Read the model definition and answer for the solid it produces. Units are mm, in the model's axes. Face numbers are marked on the shaded views. A direction names the side the tool comes from. Coordinates: 2 decimals unless noted, no trailing zeros. Write each loop counter-clockwise with the first axis right and the second up, starting at its lowest first coordinate (ties: lowest second). Pieces come first, ordered by that corner, then holes.
1) Find the intervals of material crossed by line 1 (Y direction, x = -29, z = 3.35); line 2 (Y direction, x = -24, z = 1.8); line 3 (X direction, y = -20, z = 1.9), in increasing order.
2) The part is cut by section D-D (x = -33). Determine the outline of the cut face in (y, z).
3) The part is cut by section A-A (x = -24). Determine the outline of the cut face in (y, z), then the cut area to 3 significant figures.
4) Determine the mould class of the marked faces 1, 2 and 3 for opening direction X: +X half, -X half, draft (parallel to the pull), parting line (faces both ways), or undercut.
5) The part is cut by section B-B (y = -2). Determine the outline of the cut face in (x, z).
6) Each of these flat-tipped pins is pushed along its axis until it touches: pin 1 Ø2 at (x, z) = (-41, 2) entering from +Y; pin 2 Ø1.2 at (x, z) = (-40, 1.5) entering from -Y; pin 3 Ø1.2 at (y, z) = (-40, 2.5) entering from -X. Where does it stop, or does it pass through?
7) Which of the six approach directions +Z, -Z, +X, -X, +Y, -Y give full straight-line access (tool end or side, diameter ignored) to the marked faces 4, 5 and 6?
8) The part is cut by section C-C (z = 2.75). Give the number of separate pieces and of enclosed holes in the cut face, then the cut area to 3 significant figures.
Autodesk Inventor part; units mm, degrees
ref_plane "YZ Plane" through (0, 0, 0) normal (1, 0, 0) x (0, 1, 0)
ref_plane "XZ Plane" through (0, 0, 0) normal (0, 1, 0) x (-1, 0, 0)
ref_plane "XY Plane" through (0, 0, 0) normal (0, 0, 1) x (1, 0, 0)
sketch "Sketch1" plane through (0, 0, 0) normal (0, 0, 1) x (1, 0, 0)
  line L0 (-49.5875, 0) -> (0, 0)
  line L1 (0, 0) -> (0, -41.788)
  line L2 (0, -41.788) -> (-49.5875, -41.788)
  line L3 (-49.5875, -41.788) -> (-49.5875, 0)
  circle A0 centre (-24, -20.894) radius 3.4749
  circle A1 centre (-24, -20.894) radius 4
  point P0 (0, 0)
  dimension "d0" = 8
extrude "Extrusion1" add sketch "Sketch1" along normal blind 4 contours L0 L1 L2 L3
fillet "Fillet1" radius 3.175 2 edges at (-49.5875, 0, 2) (-49.5875, -41.788, 2)
sketch "Sketch2" plane through (0, 0, 4) normal (0, 0, 1) x (1, 0, 0)
  line L0 (-42.7117, -37.788) -> (-36.7117, -37.788) construction
  line L1 (-42.7117, -37.788) -> (-42.7117, -41.788) construction
  line L2 (-36.7117, -41.788) -> (-42.7117, -41.788) construction
  line L3 (-36.7117, -37.788) -> (-36.7117, -41.788) construction
  line L4 (-21.5117, -37.788) -> (-15.5117, -37.788) construction
  line L5 (-21.5117, -37.788) -> (-21.5117, -41.788) construction
  line L6 (-15.5117, -41.788) -> (-21.5117, -41.788) construction
  line L7 (-15.5117, -37.788) -> (-15.5117, -41.788) construction
  line L8 (-21.5117, 0) -> (-15.5117, 0) construction
  line L9 (-21.5117, 0) -> (-21.5117, -4) construction
  line L10 (-15.5117, -4) -> (-21.5117, -4) construction
  line L11 (-15.5117, 0) -> (-15.5117, -4) construction
  line L12 (-42.7117, 0) -> (-36.7117, 0) construction
  line L13 (-42.7117, 0) -> (-42.7117, -4) construction
  line L14 (-36.7117, -4) -> (-42.7117, -4) construction
  line L15 (-36.7117, 0) -> (-36.7117, -4) construction
  line L16 (-27.4117, -4) -> (-30.8117, -4) construction
  line L17 (-27.4117, 0) -> (-27.4117, -4) construction
  line L18 (-30.8117, 0) -> (-27.4117, 0) construction
  line L19 (-30.8117, 0) -> (-30.8117, -4) construction
  line L20 (-27.4117, -41.788) -> (-30.8117, -41.788) construction
  line L21 (-27.4117, -37.788) -> (-27.4117, -41.788) construction
  line L22 (-30.8117, -37.788) -> (-27.4117, -37.788) construction
  line L23 (-30.8117, -37.788) -> (-30.8117, -41.788) construction
  line L24 (-42.9117, -41.988) -> (-42.9117, -37.588)
  line L25 (-42.9117, -37.588) -> (-36.5117, -37.588)
  line L26 (-36.5117, -37.588) -> (-36.5117, -41.988)
  line L27 (-36.5117, -41.988) -> (-42.9117, -41.988)
  line L28 (-21.7117, -41.988) -> (-21.7117, -37.588)
  line L29 (-21.7117, -37.588) -> (-15.3117, -37.588)
  line L30 (-15.3117, -37.588) -> (-15.3117, -41.988)
  line L31 (-15.3117, -41.988) -> (-21.7117, -41.988)
  line L32 (-42.9117, -4.2) -> (-42.9117, 0.2)
  line L33 (-42.9117, 0.2) -> (-36.5117, 0.2)
  line L34 (-36.5117, 0.2) -> (-36.5117, -4.2)
  line L35 (-36.5117, -4.2) -> (-42.9117, -4.2)
  line L36 (-21.7117, -4.2) -> (-21.7117, 0.2)
  line L37 (-21.7117, 0.2) -> (-15.3117, 0.2)
  line L38 (-15.3117, 0.2) -> (-15.3117, -4.2)
  line L39 (-15.3117, -4.2) -> (-21.7117, -4.2)
  circle A0 centre (-29.1117, -39.788) radius 1.6
  circle A1 centre (-29.1117, -2) radius 1.6
  point P0 (0, 0)
  dimension "d4" = 0.2
  dimension "d5" = 0.2
  dimension "d6" = 0.2
  dimension "d7" = 0.2
  dimension "d8" = 3.2
  dimension "d9" = 3.2
extrude "Extrusion2" cut sketch "Sketch2" against normal blind 4
sketch "Sketch3" plane through (0, 0, 0) normal (0, 0, -1) x (-1, 0, 0)
  circle A0 centre (27.6419, -12.6638) radius 1.5 construction
  circle A1 centre (29.3066, -28.1631) radius 1.5 construction
  circle A2 centre (15.0515, -21.8552) radius 1.5 construction
  circle A3 centre (24, -20.894) radius 3.4749 construction
  circle A4 centre (24, -20.894) radius 9 construction
  circle A5 centre (33, -20.894) radius 1.5
  circle A6 centre (19.5, -28.6882) radius 1.5
  circle A7 centre (19.5, -13.0998) radius 1.5
  point P0 (0, 0)
  dimension "d12" = 3
  dimension "d15" = 360
extrude "Extrusion3" cut sketch "Sketch3" against normal blind 4
properties part number "Wiper nut holder"
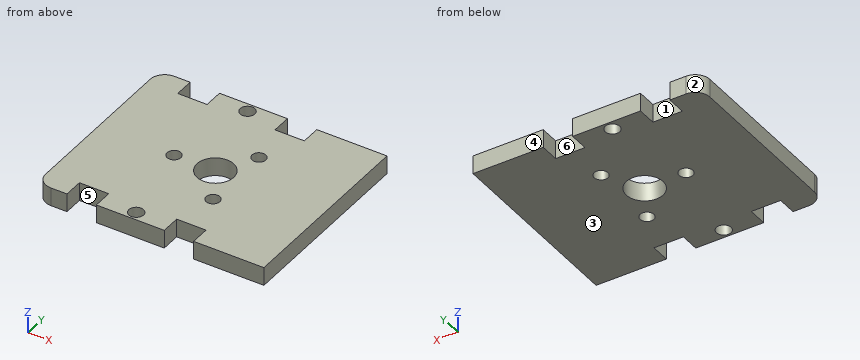
Reported:
1. line 1: y = -41.79 to -41.38, -38.19 to -3.6, -0.4 to 0
1. line 2: y = -41.79 to -24.89, -16.89 to 0
1. line 3: x = -49.59 to -34.2, -31.8 to -27.9, -20.1 to 0
2. outline: (-41.79, 0) - (-22.39, 0) - (-22.39, 4) - (-41.79, 4) - close; (-19.39, 0) - (0, 0) - (0, 4) - (-19.39, 4) - close
3. outline: (-41.79, 0) - (-24.89, 0) - (-24.89, 4) - (-41.79, 4) - close; (-16.89, 0) - (0, 0) - (0, 4) - (-16.89, 4) - close
3. area: 135 mm2
4. face 1: undercut
4. face 2: -X half
4. face 3: draft
5. outline: (-49.36, 0) - (-42.91, 0) - (-42.91, 4) - (-49.36, 4) - close; (-36.51, 0) - (-30.71, 0) - (-30.71, 4) - (-36.51, 4) - close; (-27.51, 0) - (-21.71, 0) - (-21.71, 4) - (-27.51, 4) - close; (-15.31, 0) - (0, 0) - (0, 4) - (-15.31, 4) - close
6. pin 1: stops at y = -4.2
6. pin 2: stops at y = -37.59
6. pin 3: stops at x = -49.49
7. face 4: +Z, -Z, +X, -X, +Y
7. face 5: +Z, -Z, -Y
7. face 6: +Z, -Z, +Y
8. separate pieces: 1
8. enclosed holes: 6
8. area: 1,870 mm2
